```python
from build123d import *

# Parameters (mm, degrees)
EXTRUDE_1_DEPTH       = 2
HOLE_WIZARD_4_0_4_1_D = 4
FILLET_1_R            = 5
FILLET_2_R            = 5
HOLE_WIZARD_4_0_4_2_D = 4


with BuildPart() as part:
    # 草圖1 → 填料-伸長1 (new body)
    with BuildSketch(Plane(origin=(0, 0, 0), x_dir=(1, 0, 0), z_dir=(0, 1, 0))):
        Polygon((0, 0), (18, 0), (18, 38), (38, 38), (38, 0), (56, 0), (56, -20), (0, -20), align=None)
    extrude(amount=EXTRUDE_1_DEPTH)

    # Ø4.0 (4) 直徑孔1 (through all)
    with Locations(Plane(origin=(0, 0, 0), x_dir=(-1, 0, 0), z_dir=(0, -1, 0))):
        with Locations((-28, 30), (-28, 10), (-28, -10), (-8, -10), (-48, -10)):
            Hole(HOLE_WIZARD_4_0_4_1_D / 2)

    # 圓角1
    fillet_1_edges = [part.edges().sort_by_distance(p)[0] for p in [
        (0, 1, 0),
        (18, 1, -38),
        (38, 1, -38),
        (56, 1, 0),
        (56, 1, 20),
        (0, 1, 20),
    ]]
    fillet(fillet_1_edges, radius=FILLET_1_R)

    # 圓角2
    fillet_2_edges = [part.edges().sort_by_distance(p)[0] for p in [
        (18, 1, 0),
        (38, 1, 0),
    ]]
    fillet(fillet_2_edges, radius=FILLET_2_R)

    # Ø4.0 (4) 直徑孔2 (through all)
    with Locations(Plane(origin=(0, 0, 0), x_dir=(-1, 0, 0), z_dir=(0, -1, 0))):
        with Locations((-38, -10), (-18, -10), (-28, 20)):
            Hole(HOLE_WIZARD_4_0_4_2_D / 2)


solid = part.part
```
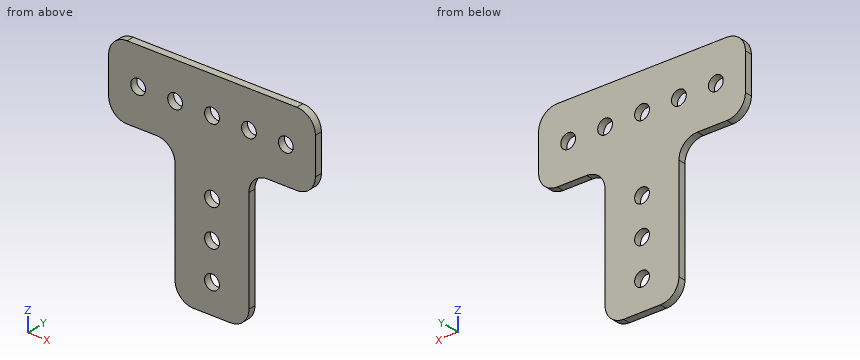
Geometry: final body of the model. Coordinates: model frame, mm. Give positions to 0.01 mm unless a question says otherwise; leave off trailing zeros. Order: outer loops, then holes, each group sorted by start corner. A loop starts at its lowest first (then second) coordinate and runs counter-clockwise, first axis right, second up. Notation, with made-up numbers: (-37, 81) -> (13, 81) arc R25 cw to (13, 119) -> close; hole circle Ø5 at (44, 54.25). An arc over 180 degrees is marked (long way). Write each question's results on one line, items separated by ' | '. Start each with the question number.
1) Section D-D (x = 28). Return loops of the section in (y, z).
2) First-contact query: pin 1 (2.5 mm diameter, centred on x = 18, z = 10, fed in from +Y); pin 2 (5 mm diameter, centred on x = 28, z = -10, fed in from +Y); pin 3 (1 mm diameter, centred on y = 1, z = -21, fed in from -X); pin 4 (0.6 mm diameter, centred on y = 0.5, z = -18, fed in from +X). Flat tips, straight axial feed; report the tip coordinate or a pass-through.
3) Section C-C (y = 1.65). Count the separate pieces of the cut face and the enclosed holes in it, then the cut area to 3 significant figures.
4) Section A-A (x = 48). Return loops of the section in (y, z).
5) Line query: line 1 (Z direction, x = 28, y = 1.5); line 2 (X direction, y = 0.5, z = 10); line 3 (X direction, y = 1.8, z = 11). Output: solid intervals per line, ascending. Write a range as from..to.
6) Section B-B (z = 10). Return loops of the section in (x, y).
Calculated:
1) outline: (0, -38) -> (2, -38) -> (2, -32) -> (0, -32) -> close; (0, -28) -> (2, -28) -> (2, -22) -> (0, -22) -> close; (0, -18) -> (2, -18) -> (2, -12) -> (0, -12) -> close; (0, -8) -> (2, -8) -> (2, 8) -> (0, 8) -> close; (0, 12) -> (2, 12) -> (2, 20) -> (0, 20) -> close
2) pin 1: through | pin 2: y = 2 | pin 3: x = 18 | pin 4: x = 38
3) separate pieces: 1 | enclosed holes: 8 | area: 1,760 mm2
4) outline: (0, 0) -> (2, 0) -> (2, 8) -> (0, 8) -> close; (0, 12) -> (2, 12) -> (2, 20) -> (0, 20) -> close
5) line 1: -38..-32, -28..-22, -18..-12, -8..8, 12..20 | line 2: 0..6, 10..16, 20..26, 30..36, 40..46, 50..56 | line 3: 0..6.27, 9.73..16.27, 19.73..26.27, 29.73..36.27, 39.73..46.27, 49.73..56
6) outline: (0, 0) -> (6, 0) -> (6, 2) -> (0, 2) -> close; (10, 0) -> (16, 0) -> (16, 2) -> (10, 2) -> close; (20, 0) -> (26, 0) -> (26, 2) -> (20, 2) -> close; (30, 0) -> (36, 0) -> (36, 2) -> (30, 2) -> close; (40, 0) -> (46, 0) -> (46, 2) -> (40, 2) -> close; (50, 0) -> (56, 0) -> (56, 2) -> (50, 2) -> close
